```python
from build123d import *

# Parameters (mm, degrees)
CROQUIS1_W              = 1
CROQUIS1_H              = 20
SALIENTE_EXTRUIR1_DEPTH = 30
CROQUIS2_W              = 4
CROQUIS2_H              = 1
SALIENTE_EXTRUIR3_DEPTH = 30
SALIENTE_EXTRUIR4_DEPTH = 1
SALIENTE_EXTRUIR5_DEPTH = 1
SALIENTE_EXTRUIR7_DEPTH = 1
NERVIO4_REACH           = 38.239
CROQUIS8_WALL_W         = 93.582555916
CROQUIS8_WALL_H         = 1
MATRIZL12_COUNT         = 9
MATRIZL12_PITCH         = 3
NERVIO5_REACH           = 38.239
CROQUIS10_WALL_W        = 93.582555916
CROQUIS10_WALL_H        = 1


with BuildPart() as part:
    # Croquis1 → Saliente-Extruir1 (new body)
    with BuildSketch(Plane(origin=(0, 0, 0), x_dir=(0, 0, -1), z_dir=(1, 0, 0))):
        with Locations((0.5, 10)):
            Rectangle(CROQUIS1_W, CROQUIS1_H)
    extrude(amount=-SALIENTE_EXTRUIR1_DEPTH)

    # Croquis2 → Saliente-Extruir3 (add)
    with BuildSketch(Plane(origin=(0, 0, 0), x_dir=(0, 0, -1), z_dir=(1, 0, 0))):
        with Locations((-2, 0.5)):
            Rectangle(CROQUIS2_W, CROQUIS2_H)
    extrude(amount=-SALIENTE_EXTRUIR3_DEPTH)

    # Croquis3 → Saliente-Extruir4 (add)
    with BuildSketch(Plane(origin=(0, 0, 0), x_dir=(0, 0, -1), z_dir=(1, 0, 0))):
        Polygon((-4, 1), (-1, 20), (0, 20), (0, 1), align=None)
    extrude(amount=-SALIENTE_EXTRUIR4_DEPTH)

    # Croquis6 → Saliente-Extruir5 (add)
    with BuildSketch(Plane.ZY.offset(30)):
        Polygon((0, 20), (1, 20), (4, 1), (0, 1), align=None)
    extrude(amount=-SALIENTE_EXTRUIR5_DEPTH)

    # Croquis7 → Saliente-Extruir7 (add)
    with BuildSketch(Plane(origin=(0, 1, 0), x_dir=(1, 0, 0), z_dir=(0, 1, 0))):
        Polygon((-30, -4), (-28.232233047, -5.767766953), (-15, -8.5), (-1.767766953, -5.767766953), (0, -4), align=None)
    extrude(amount=-SALIENTE_EXTRUIR7_DEPTH)

    # Croquis8 wall → Nervio4 (add, up to next)
    with BuildSketch(Plane(origin=(-29, 10.5, 1), x_dir=(0, 0.994505452921, -0.104684784518), z_dir=(0, 0.104684784518, 0.994505452921)), mode=Mode.PRIVATE) as nervio4_sk1:
        with Locations((0, -0.5)):
            Rectangle(CROQUIS8_WALL_W, CROQUIS8_WALL_H)
    nervio4_tool1 = extrude(nervio4_sk1.sketch, amount=-NERVIO4_REACH, mode=Mode.PRIVATE) - part.part
    nervio4 = nervio4_tool1.solids().sort_by_distance((-29, 10.5, 1))[0]
    add(nervio4)

    # MatrizL12: Nervio4 ×9
    with Locations(*[(i * MATRIZL12_PITCH, 0, 0) for i in range(1, MATRIZL12_COUNT)]):
        add(nervio4)

    # Croquis10 wall → Nervio5 (add, up to next)
    with BuildSketch(Plane(origin=(-1, 10.5, 1), x_dir=(0, 0.994505452921, -0.104684784518), z_dir=(0, -0.104684784518, -0.994505452921)), mode=Mode.PRIVATE) as nervio5_sk1:
        with Locations((0, -0.5)):
            Rectangle(CROQUIS10_WALL_W, CROQUIS10_WALL_H)
    nervio5_tool1 = extrude(nervio5_sk1.sketch, amount=NERVIO5_REACH, mode=Mode.PRIVATE) - part.part
    add(nervio5_tool1.solids().sort_by_distance((-1, 10.5, 1))[0])


solid = part.part
```
Geometry: final body of the model. Coordinates: model frame, mm. A direction names the side the tool comes from. Round coordinates to 2 decimals unless told otherwise and drop trailing zeros. Write each loop counter-clockwise with the first axis right and the second up, starting at its lowest first coordinate (ties: lowest second). Pieces come first, ordered by that corner, then holes.
Item 1: Pin query (flat end, axial travel): P1, Ø0.6, axis at x = -21.5, y = 9.5, coming from the +Z side; P2, Ø1.5, axis at y = 11.5, z = 4.5, coming from the +X side; P3, Ø10, axis at x = -18, y = 7.5, coming from the +Z side; P4, Ø4, axis at x = -21.5, z = 6.5, coming from the +Y side. Return the tip coordinate at first contact, or that it passes through.
Item 2: Section query D-D (z = 6.5). Return loops of the section in (x, y).
Item 3: Section query C-C (x = -23.75). Return loops of the section in (y, z), plus the area to 3 significant figures.
Item 4: Mould query, pull axis X, two halves, no side actions, for faces 3 (the face through (-29.1, 0.5, 4.9)), 4 (the face through (-3, 10, 0)), 5 (the face through (-29.51, 10.63, 2.48)), 6 (the face through (-13.507, 10.367, 1.014)). Classes: +X half, -X half, draft (parallel to the pull), parting line (faces both ways), or undercut.
Item 5: Material intervals for L1, parallel to X at y = 3, z = 2.75; L2, parallel to Z at x = -9, y = 14; L3, parallel to Y at x = -6, z = 0.5, sorted ascending.
Item 6: Set-up query: faces 1 (the face through (-15, 0, 3)), 2 (the face through (-29, 9, 2)). Return all of +Z, -Z, +X, -X, +Y, -Y with unobstructed straight access to the full face (end or side cutting, diameter ignored); none if empty.
Item 7: Section query B-B (x = -7.5). Return loops of the section in (y, z), plus the area to 3 significant figures.
Item 8: Section query A-A (z = 2.5). Return loops of the section in (x, y).
Completed:
1. P1: stops at z = 0
1. P2: passes through
1. P3: stops at z = 1.83
1. P4: stops at y = 1
2. outline: (-24.69, 0) - (-5.31, 0) - (-5.31, 1) - (-24.69, 1) - close
3. outline: (0, -1) - (20, -1) - (20, 0) - (1, 0) - (1, 6.69) - (0, 6.69) - close
3. area: 26.7 mm2
4. face 3: -X half
4. face 4: undercut
4. face 5: draft
4. face 6: undercut
5. L1: x = -30 to -29, -1 to 0
5. L2: z = -1 to 0
5. L3: y = 0 to 1
6. face 1: +Z, -Z, +X, -X, -Y
6. face 2: +Z, +Y
7. outline: (0, -1) - (20, -1) - (20, 0) - (1, 2) - (1, 6.95) - (0, 6.95) - close
7. area: 46.0 mm2
8. outline: (-30, 0) - (0, 0) - (0, 10.5) - (-1, 10.5) - (-1, 1) - (-29, 1) - (-29, 10.5) - (-30, 10.5) - close
